Here's how the part is built. I have some questions about the finished solid (model axes, mm). Face numbers are marked on the shaded views. A direction names the side the tool comes from. Round coordinates to 2 decimals unless told otherwise and drop trailing zeros. Write each loop counter-clockwise with the first axis right and the second up, starting at its lowest first coordinate (ties: lowest second). Pieces come first, ordered by that corner, then holes. Notation, with made-up numbers: (-18, -6.5) - (41, -6.5) arc R10 ccw to (41, 6.5) - close; hole circle Ø9 at (46.5, -18.5). An arc over 180 degrees is marked (long way). Return JSON: item names as keys, results as strings. Group by question number.
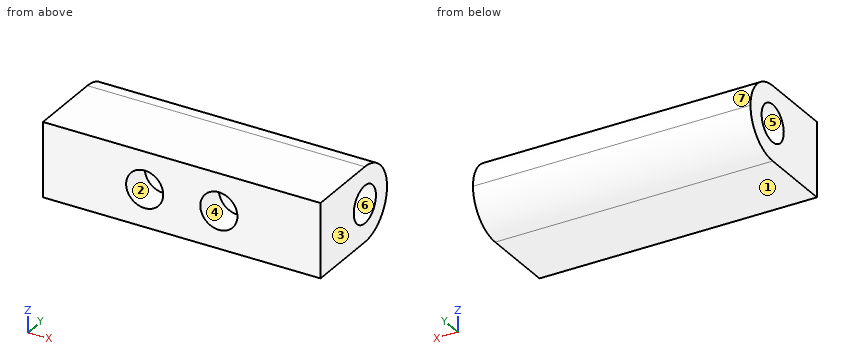
```python
from build123d import *

# Parameters (mm, degrees)
SKETCH1_W                 = 37.4
SKETCH1_H                 = 10
BOSS_EXTRUDE1_DEPTH       = 15
FILLET1_R                 = 5
F_1_0MM_DOWEL_HOLE1_D     = 5
F_1_0MM_DOWEL_HOLE1_DEPTH = 4.2
F_1_0MM_DOWEL_HOLE1_TIP   = 1.502151548


with BuildPart() as part:
    # Sketch1 → Boss-Extrude1 (new body)
    with BuildSketch(Plane(origin=(0, 0, 0), x_dir=(1, 0, 0), z_dir=(0, 1, 0))):
        Rectangle(SKETCH1_W, SKETCH1_H)
    extrude(amount=BOSS_EXTRUDE1_DEPTH)

    # Fillet1
    fillet1_edges = [part.edges().sort_by_distance(p)[0] for p in [
        (0, 15, -5),
        (0, 15, 5),
    ]]
    fillet(fillet1_edges, radius=FILLET1_R - 0.0001)  # a hair under: the kernel refuses the full size

    # Sketch11 → CBORE for M5 Hex Head Bolt2 (revolve, cut)
    with BuildSketch(Plane(origin=(-18.7, 10, 0), x_dir=(0, 0, 1), z_dir=(0, 1, 0))):
        Polygon((0, 0), (0, 11.351936393), (2.25, 10), (2.25, 8), (2.5, 8), (2.5, 0), align=None)
    cbore_for_m5_hex_head_bolt2 = revolve(axis=Axis((-25.05, 10, 0), (1, 0, 0)), mode=Mode.SUBTRACT)

    # Mirror1: CBORE for M5 Hex Head Bolt2 across plane
    add(cbore_for_m5_hex_head_bolt2.mirror(Plane(origin=(0, 0, 0), x_dir=(0, 0, 1), z_dir=(1, 0, 0))), mode=Mode.SUBTRACT)

    # Ø1.0mm Dowel Hole1
    with Locations(Plane(origin=(0, 0, 0), x_dir=(-1, 0, 0), z_dir=(0, -1, 0))):
        with Locations((-5, 0), (5, 0)):
            Hole(F_1_0MM_DOWEL_HOLE1_D / 2, depth=F_1_0MM_DOWEL_HOLE1_DEPTH)
            with Locations((0, 0, -(F_1_0MM_DOWEL_HOLE1_DEPTH + F_1_0MM_DOWEL_HOLE1_TIP / 2))):  # 118° drill point
                Cone(0, F_1_0MM_DOWEL_HOLE1_D / 2, F_1_0MM_DOWEL_HOLE1_TIP, mode=Mode.SUBTRACT)


solid = part.part
```
1) I need wall thicknesses on line 1 along Z through (x, y) = (-14.25, 10); line 2 along Y through (x, z) = (-17, 0); line 3 along Z through (x, y) = (9.65, 10). Which ranges of each line are inside material? Lowest first, please.
2) Imagine slicing it at B-B (y = 3.5). Please give me the cut outline in (x, z), plus the area to 3 significant figures.
3) Will these pins go through, and if not, where does the flat tip stop? pin 1 Ø1.5 at (y, z) = (9, -1) entering from -X; pin 2 Ø3 at (x, z) = (-6.5, 2) entering from +Y; pin 3 Ø3 at (x, z) = (4.5, -3.5) entering from +Y.
4) For the marked faces 5, 6 and 7, which set-ups out of +Z, -Z, +X, -X, +Y, -Y let a thin tool reach every point of the face, with its end or its side?
5) If we mould it in two halves opening along X, with no side actions, what happens to the marked faces 1, 2, 3 and 4? For each: released by +X, released by -X, zero draft, split by the parting line, or undercut.
Results found:
{
 "1": {"line 1": "z = -5 to -2.5, 2.5 to 5", "line 2": "y = 0 to 7.5, 12.5 to 15", "line 3": "z = -5 to -2.25, 2.25 to 5"},
 "2": {"outline": "(-18.7, -5) - (18.7, -5) - (18.7, 5) - (-18.7, 5) - close; hole circle Ø5 at (-5, 0); hole circle Ø5 at (5, 0)", "area": "335 mm²"},
 "3": {"pin 1": "stops at x = -8.65", "pin 2": "stops at y = 14.97", "pin 3": "stops at y = 14.58"},
 "4": {"face 5": "-X", "face 6": "+X", "face 7": "+Z, +X, -X, +Y"},
 "5": {"face 1": "zero draft", "face 2": "undercut", "face 3": "released by +X", "face 4": "undercut"}
}
